Part model, mm, in its own coordinate system. Face numbers are marked on the shaded views. A direction names the side the tool comes from. Give positions to 0.01 mm unless a question says otherwise; leave off trailing zeros. Write each loop counter-clockwise with the first axis right and the second up, starting at its lowest first coordinate (ties: lowest second). Pieces come first, ordered by that corner, then holes. Notation, with made-up numbers: M 36,2 L 67,2 A19 cw 67,24 Z; hole C 48,-37 d6. An arc over 180 degrees is marked long. Use CSV: the item, a comma, the result in double quotes. Start each with the question number.
Item 1: Cut at A-A (z = -37.5). List the corners of the cut face in (x, y), then the cut area to 3 significant figures.
Item 2: Which spindle directions (+Z, -Z, +X, -X, +Y, -Y) get a long thin tool onto all of the face, cutting with end or side? Do the marked faces 1 and 2. Say none if no direction does.
Item 3: Cut at B-B (z = -20). List the corners of the cut face in (x, y).
Item 4: Drill centre lines: line 1 (X direction, y = 1.85, z = -19.5); line 2 (Y direction, x = 3.5, z = -37); line 3 (Z direction, x = 24, y = 0.9). Where is each one in solid material? Low to high. Write a range as [from, to].
Item 5: Pin check, flat tips, straight feed: pin 1 (1.1 mm diameter, centred on x = 1.5, y = 1, fed in from -Z); pin 2 (8.5 mm diameter, centred on x = 26.5, z = -36.5, fed in from +Y). Stop position of each tip, or through.
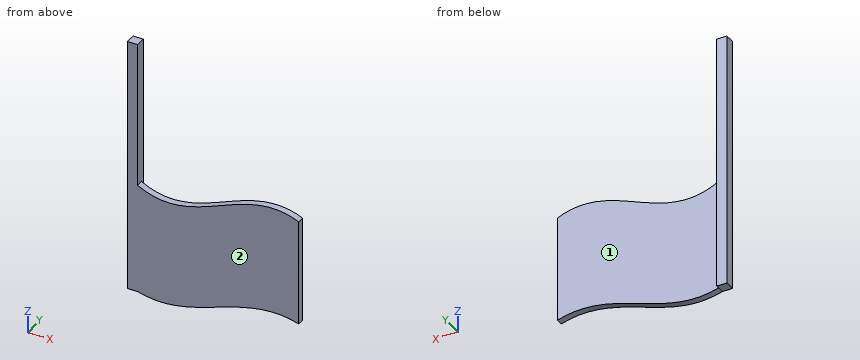
from build123d import *

# Parameters (mm, degrees)
SKETCH1_W           = 2.2
SKETCH1_H           = 55
BOSS_EXTRUDE1_DEPTH = 2.2
BOSS_EXTRUDE2_DEPTH = 1.5


with BuildPart() as part:
    # Sketch1 → Boss-Extrude1 (new body)
    with BuildSketch(Plane(origin=(0, 0, 0), x_dir=(1, 0, 0), z_dir=(0, 1, 0))):
        with Locations((1.1, 27.5)):
            Rectangle(SKETCH1_W, SKETCH1_H)
    extrude(amount=BOSS_EXTRUDE1_DEPTH)

    # Sketch2 → Boss-Extrude2 (add)
    with BuildSketch(Plane(origin=(0, 0, 0), x_dir=(1, 0, 0), z_dir=(0, 1, 0))):
        with BuildLine():
            Line((36.906195037, 51.326121053), (36.906195037, 28.571653378))
            add(Edge.make_bspline(
                [(2.2, 31.323116725), (14.559505751, 38.154017268), (24.656914199, 23.036255891), (36.906195037, 28.571653378)],
                knots=[0, 0, 0, 0, 1, 1, 1, 1], degree=3))
            Line((2.2, 31.323116725), (2.2, 55))
            add(Edge.make_bspline(
                [(2.2, 55), (14.296538577, 58.763817037), (24.50579778, 47.343941309), (36.906195037, 51.326121053)],
                knots=[0, 0, 0, 0, 1, 1, 1, 1], degree=3))
        make_face()
    extrude(amount=BOSS_EXTRUDE2_DEPTH)


solid = part.part
Worked answers:
1,outline,"M 0,0 L 36.91,0 L 36.91,1.5 L 2.2,1.5 L 2.2,2.2 L 0,2.2 Z"
1,area,"56.9 mm^2"
2,face 1,"+Z, -Z, +X, +Y"
2,face 2,"+Z, -Z, +X, -X, -Y"
3,outline,"M 0,0 L 2.2,0 L 2.2,2.2 L 0,2.2 Z"
4,line 1,"x = [0, 2.2]"
4,line 2,"y = [0, 1.5]"
4,line 3,"z = [-51.64, -28.74]"
5,pin 1,"stops at z = -55"
5,pin 2,"stops at y = 1.5"
